Geometry check sheet. Reference: the model listing, model coordinates, mm. Round coordinates to 2 decimals unless told otherwise and drop trailing zeros. Order: outer loops, then holes, each group sorted by start corner. A loop starts at its lowest first (then second) coordinate and runs counter-clockwise, first axis right, second up. Notation, with made-up numbers: (80, -32) - (120, -32) arc R18 cw to (120, -20) - close; hole circle Ø7 at (69, -14.5). An arc over 180 degrees is marked (long way). Write each question's results on one line, items separated by ' | '.
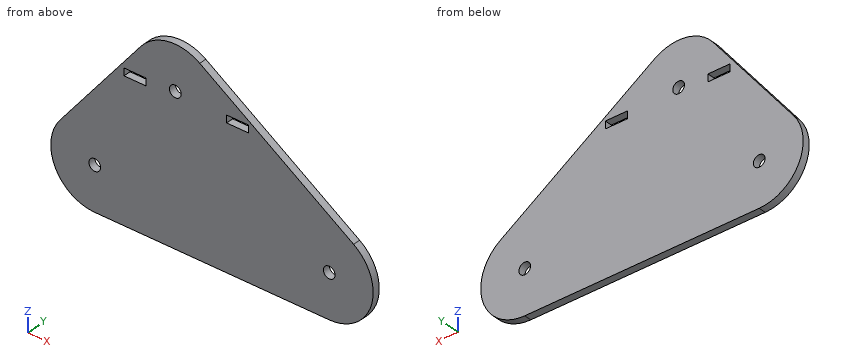
```python
from build123d import *

# Parameters (mm, degrees)
F0_R     = 4
F1_DEPTH = 5
F2_W     = 15
F2_H     = 5
F3_DEPTH = 5


with BuildPart() as f1:
    # F0 (on Front) → F1 (new body)
    with BuildSketch(Plane.XZ):
        with BuildLine():
            Line((-23.58955, 88.534647), (-78.58955, 18.534647))
            ThreePointArc((-78.58955, 18.534647), (-81.98184, -13.114126), (-55, -30))
            Line((-55, -30), (105, -30))
            ThreePointArc((105, -30), (133.712761, -8.693524), (121.641006, 24.961509))
            Line((121.641006, 24.961509), (16.641006, 94.961509))
            ThreePointArc((16.641006, 94.961509), (-4.732516, 99.62437), (-23.58955, 88.534647))
        make_face()
        with Locations((-55, 0)):
            Circle(F0_R, mode=Mode.SUBTRACT)
        with Locations((105, 0)):
            Circle(F0_R, mode=Mode.SUBTRACT)
        with Locations((0, 70)):
            Circle(F0_R, mode=Mode.SUBTRACT)
    extrude(amount=F1_DEPTH)

    # F2 (on face) → F3 (cut)
    with BuildSketch(Plane.XZ.offset(5)):
        with Locations((-27.5, 67.5)):
            Rectangle(F2_W, F2_H)
        with Locations((42.5, 67.5)):
            Rectangle(F2_W, F2_H)
    extrude(amount=-F3_DEPTH, mode=Mode.SUBTRACT)


solid = f1.part
```
(1) Section check C-C (y = -3.35). Record the cut outline in (x, z).
Answers follow:
outline: (-78.59, 18.53) arc R30 ccw to (-55, -30) - (105, -30) arc R30 ccw to (121.64, 24.96) - (16.64, 94.96) arc R30 ccw to (-23.59, 88.53) - close; hole circle Ø8 at (-55, 0); hole (-35, 65) - (-20, 65) - (-20, 70) - (-35, 70) - close; hole circle Ø8 at (0, 70); hole (35, 65) - (50, 65) - (50, 70) - (35, 70) - close; hole circle Ø8 at (105, 0)
(2) Section check D-D (x = -31). Record the cut outline in (y, z).
Answers follow:
outline: (-5, -30) - (0, -30) - (0, 65) - (-5, 65) - close; (-5, 70) - (0, 70) - (0, 79.1) - (-5, 79.1) - close
(3) Section check A-A (z = 0). Record the cut outline in (x, y), then the cut area to 3 significant figures.
Answers follow:
outline: (-85, -5) - (-59, -5) - (-59, 0) - (-85, 0) - close; (-51, -5) - (101, -5) - (101, 0) - (-51, 0) - close; (109, -5) - (135, -5) - (135, 0) - (109, 0) - close | area: 1,020 mm²
(4) Depth check by flat-ended pin: pin 1 Ø2.5 at (x, y) = (-27.5, -3) entering from +Z; pin 2 Ø1.5 at (y, z) = (-3.5, 67) entering from +X; pin 3 Ø3 at (y, z) = (-1.5, 29.5) entering from -X; pin 4 Ø6.5 at (x, z) = (-55, 0) entering from +Y. Enter the tip coordinate at first touch or a pass-through.
Answers follow:
pin 1: z = 85.15 | pin 2: x = 59.71 | pin 3: x = -71.15 | pin 4: through
(5) Section check B-B (x = 0). Record the cut outline in (y, z).
Answers follow:
outline: (-5, -30) - (0, -30) - (0, 66) - (-5, 66) - close; (-5, 74) - (0, 74) - (0, 100) - (-5, 100) - close
(6) Material ranges on line 1 (Z direction, x = 0, y = -3.3); line 2 (X direction, y = -3.9, z = -2.5); line 3 (X direction, y = -4, z = 67), recorded low to high.
Answers follow:
line 1: -30 to 66, 74 to 100 | line 2: -84.9 to -58.12, -51.88 to 101.88, 108.12 to 134.9 | line 3: -40.51 to -35, -20 to -2.65, 2.65 to 35, 50 to 58.58
